Print and shaded views of the part. All mm, measured from the part's lowest x, y and z. Round coordinates to 2 decimals unless told otherwise and drop trailing zeros. Order: outer loops, then holes, each group sorted by start corner. A loop starts at its lowest first (then second) coordinate and runs counter-clockwise, first axis right, second up. Notation, with made-up numbers: M -34,46.5 L -5,46.5 A31 ccw -5,79.5 Z; hole C -30,4 d5. An arc over 180 degrees is marked long. Write each question's results on one line, items separated by ' | '. Start each with the question number.
1. Band-saw the part on A-A, the plane x = 6.35. List the corners of the cut face in (y, z) (3 decimals).
2. Band-saw the part on B-B, the plane z = 17. List the corners of the cut face in (x, y) (3 decimals), then the cut area to 3 significant figures.
3. Band-saw the part on D-D, the plane x = 72. List the corners of the cut face in (y, z) (3 decimals), then the cut area to 3 significant figures.
4. Probe L1, parallel to X at y = 2.45, z = 28.5; L2, parallel to Z at x = 18.5, y = 0.8 (3 decimals); L3, parallel to X at y = 0.95, z = 26.5. List the from-to ranges inside material, lowest first. Write a range as [from, to].
5. Drop flat-ended pins along their axis: pin 1 Ø1 at (y, z) = (1.5, 7) entering from -X; pin 2 Ø8 at (x, z) = (6.35, 28.5) entering from +Y (3 decimals); pin 3 Ø4.5 at (x, z) = (76.05, 28.5) entering from +Y; pin 4 Ø1 at (y, z) = (1, 11) entering from +X. Give the stop position or say it passes through.
6. Band-saw the part on C-C, the plane y = 2.1. Give the number of separate pieces and of enclosed holes in the cut face, then the cut area to 3 significant figures.
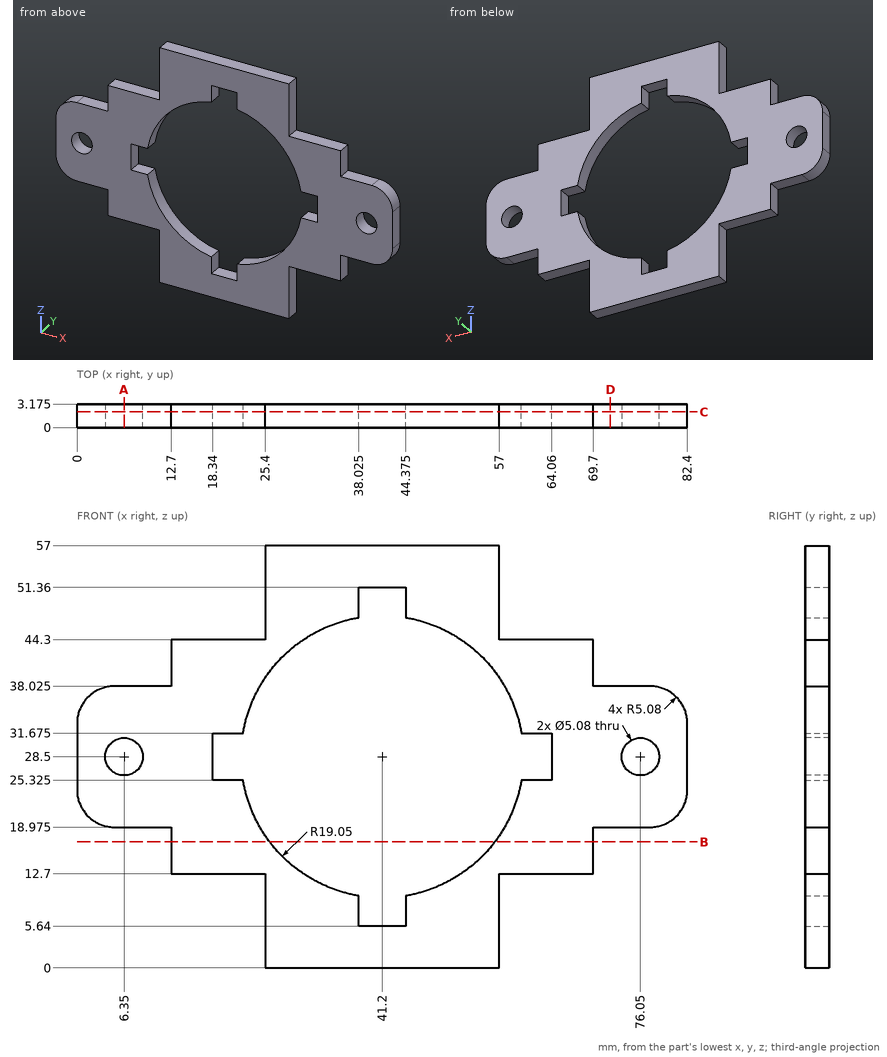
Solution:
1) outline: M 0,18.975 L 3.175,18.975 L 3.175,25.96 L 0,25.96 Z; M 0,31.04 L 3.175,31.04 L 3.175,38.025 L 0,38.025 Z
2) outline: M 12.7,0 L 26.013,0 L 26.013,3.175 L 12.7,3.175 Z; M 56.387,0 L 69.7,0 L 69.7,3.175 L 56.387,3.175 Z | area: 84.5 mm^2
3) outline: M 0,18.975 L 3.175,18.975 L 3.175,38.025 L 0,38.025 Z | area: 60.5 mm^2
4) L1: [0, 3.81], [8.89, 18.34], [64.06, 73.51], [78.59, 82.4] | L2: [12.7, 25.325], [31.675, 44.3] | L3: [0, 4.78], [7.92, 18.34], [64.06, 74.48], [77.62, 82.4]
5) pin 1: x = 25.4 | pin 2: y = 3.175 | pin 3: through | pin 4: x = 57
6) separate pieces: 1 | enclosed holes: 3 | area: 1,790 mm^2
